Read the model definition and answer for the solid it produces. Units are mm, in the model's axes. A direction names the side the tool comes from. Give positions to 0.01 mm unless a question says otherwise; leave off trailing zeros. Loops run counter-clockwise (first coordinate to the right, second up) from the corner with the lowest first, then second, coordinate; pieces in that order, holes last. Notation, with made-up numbers: (54, 70.5) -> (85, 70.5) arc R23 cw to (85, 78.5) -> close; hole circle Ø8 at (79.25, -7). An arc over 180 degrees is marked (long way). Write each question's results on one line, items separated by ' | '. Start each with the question number.
Item 1: Section B-B on z = 3 is taken. Write down the section's boundary in (x, y), and give its area (3 significant figures).
Item 2: Which of the six approach directions +Z, -Z, +X, -X, +Y, -Y give full straight-line access (tool end or side, diameter ignored) to faces 1 (the flat face through (0, -2, 0)), 2 (the flat face through (1.305, -0.74, -1.768))?
Item 3: Find the intervals of material crossed by line 1 (Z direction, x = -0.2, y = -0.2); line 2 (Y direction, x = -0.1, z = 12), in increasing order.
Item 4: Section A-A on x = 0 is taken. Write down the section's boundary in (y, z), and give its area (3 significant figures).
Item 5: Determine the mould class of faces 3 (the cylindrical face through (0.54, -2.44, -1.23)), 4 (the flat face through (0, 1.5, -2)), 5 (the flat face through (0, 0, 14)) for opening direction X: +X half, -X half, draft (parallel to the pull), parting line (faces both ways), or undercut.
Item 6: Each of these flat-tipped pins is pushed along its axis until it touches: P1, Ø1.5, axis at y = 1, z = 1, coming from the -X side; P2, Ø1.5, axis at x = -0.5, y = -0.5, coming from the -Z side; P3, Ø0.5, axis at x = 0.5, z = -1.5, coming from the -Y side. Where does it stop, or does it pass through?
```python
from build123d import *

# Parameters (mm, degrees)
ESQUISSE1_R             = 1.5
BASE_EXTRUSION_DEPTH    = 14
CHANFREIN1_SIZE         = 0.5
ESQUISSE2_R             = 2.5
BOSS_EXTRU_1_DEPTH      = 3
CONG_1_R                = 0.5
ENL_V_MAT_EXTRU_1_DEPTH = 2.5


with BuildPart() as part:
    # Esquisse1 → Base-Extrusion (new body)
    with BuildSketch(Plane.XY):
        Circle(ESQUISSE1_R)
    extrude(amount=BASE_EXTRUSION_DEPTH)

    # Chanfrein1
    chanfrein1_edges = [part.edges().sort_by_distance(p)[0] for p in [
        (-1.5, 0, 14),
    ]]
    chamfer(chanfrein1_edges, length=CHANFREIN1_SIZE)

    # Esquisse2 → Boss.-Extru.1 (add)
    with BuildSketch(Plane(origin=(0, 0, 0), x_dir=(-1, 0, 0), z_dir=(0, 0, -1))):
        Circle(ESQUISSE2_R)
    extrude(amount=BOSS_EXTRU_1_DEPTH)

    # Congé1
    cong_1_edges = [part.edges().sort_by_distance(p)[0] for p in [
        (2.5, 0, -3),
    ]]
    fillet(cong_1_edges, radius=CONG_1_R)

    # Esquisse3 → Enlèv. mat.-Extru.1 (cut)
    with BuildSketch(Plane(origin=(0, 0, -3), x_dir=(-1, 0, 0), z_dir=(0, 0, -1))):
        Polygon((1.732050808, 0), (0.866025404, 1.5), (-0.866025404, 1.5), (-1.732050808, 0), (-0.866025404, -1.5), (0.866025404, -1.5), align=None)
    extrude(amount=-ENL_V_MAT_EXTRU_1_DEPTH, mode=Mode.SUBTRACT)


solid = part.part
```
Findings:
1) outline: circle Ø3 at (0, 0) | area: 7.07 mm2
2) face 1: +Z | face 2: -Z
3) line 1: -0.5 to 14 | line 2: -1.5 to 1.5
4) outline: (-2.5, -2.5) arc R0.5 ccw to (-2, -3) -> (-1.5, -3) -> (-1.5, -0.5) -> (1.5, -0.5) -> (1.5, -3) -> (2, -3) arc R0.5 ccw to (2.5, -2.5) -> (2.5, 0) -> (1.5, 0) -> (1.5, 13.5) -> (1, 14) -> (-1, 14) -> (-1.5, 13.5) -> (-1.5, 0) -> (-2.5, 0) -> close | area: 49.1 mm2
5) face 3: parting line | face 4: undercut | face 5: draft
6) P1: x = -1.48 | P2: z = -0.5 | P3: y = -2.49
